Work out the finished part from the listing and answer in its coordinate system (mm). Face numbers are marked on the shaded views. A direction names the side the tool comes from. Give positions to 0.01 mm unless a question says otherwise; leave off trailing zeros. Write each loop counter-clockwise with the first axis right and the second up, starting at its lowest first coordinate (ties: lowest second). Pieces come first, ordered by that corner, then holes. Notation, with made-up numbers: (38, 40) -> (85, 40) arc R27 ccw to (85, 62) -> close; hole circle Ø6 at (12, 15.25). An arc over 180 degrees is marked (long way). Write item = value, one per line. Start each with the question number.
from build123d import *

# Parameters (mm, degrees)
SKETCH1_W           = 25.4
SKETCH1_H           = 50.8
SKETCH1_W_2         = 20.32
SKETCH1_H_2         = 45.72
BOSS_EXTRUDE1_DEPTH = 139.7
SKETCH2_R           = 2.032
CUT_EXTRUDE1_DEPTH  = 150.191219581
SKETCH3_R           = 2.032
SKETCH3_R_2         = 14.605
SKETCH3_R_3         = 3.302
CUT_EXTRUDE2_DEPTH  = 145.244271983


with BuildPart() as part:
    # Sketch1 → Boss-Extrude1 (new body)
    with BuildSketch(Plane.XY):
        Rectangle(SKETCH1_W, SKETCH1_H)
        Rectangle(SKETCH1_W_2, SKETCH1_H_2, mode=Mode.SUBTRACT)
    extrude(amount=BOSS_EXTRUDE1_DEPTH)

    # Sketch2 → Cut-Extrude1 (cut, through all)
    with BuildSketch(Plane(origin=(0, 25.4, 0), x_dir=(1, 0, 0), z_dir=(0, 1, 0))):
        Circle(SKETCH2_R)
        with Locations(Location((0, -25.4, 0), (0, 0, 270))):
            Circle(SKETCH2_R)
        with Locations(Location((0, -50.8, 0), (0, 0, 270))):
            Circle(SKETCH2_R)
        with Locations(Location((0, -76.2, 0), (0, 0, 270))):
            Circle(SKETCH2_R)
        with Locations(Location((0, -101.6, 0), (0, 0, 270))):
            Circle(SKETCH2_R)
        with Locations(Location((0, -127, 0), (0, 0, 270))):
            Circle(SKETCH2_R)
        with Locations((0, -152.4)):
            Circle(SKETCH2_R)
        with Locations((0, -177.8)):
            Circle(SKETCH2_R)
        with Locations((0, -203.2)):
            Circle(SKETCH2_R)
        with Locations((0, -228.6)):
            Circle(SKETCH2_R)
    extrude(amount=-CUT_EXTRUDE1_DEPTH, mode=Mode.SUBTRACT)

    # Sketch3 → Cut-Extrude2 (cut, through all)
    with BuildSketch(Plane.ZY.offset(12.7)):
        with Locations((133.35, 19.05)):
            Circle(SKETCH3_R)
        with Locations((95.25, -19.05)):
            Circle(SKETCH3_R)
        with Locations((114.3, 0)):
            Circle(SKETCH3_R_2)
        with Locations((12.7, 12.7)):
            Circle(SKETCH3_R_3)
        with Locations((38.1, 12.7)):
            Circle(SKETCH3_R_3)
        with Locations((38.1, -12.7)):
            Circle(SKETCH3_R_3)
        with Locations((12.7, -12.7)):
            Circle(SKETCH3_R_3)
    extrude(amount=-CUT_EXTRUDE2_DEPTH, mode=Mode.SUBTRACT)


solid = part.part
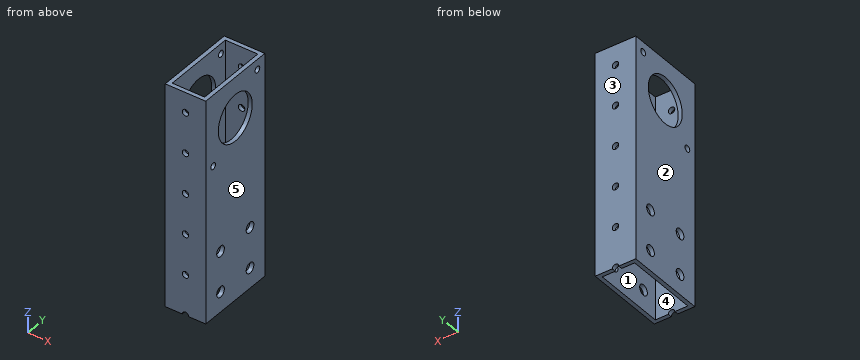
(1) Determine the mould class of the marked faces 1, 2 and 3 for opening direction X: pulls with the +X half, pulls with the -X half, needs draft (parallel to the pull), parting line crosses it, or undercut.
(2) A cutting plane is placed at D-D, the plane y = -19.05. Write down the section's boundary in (x, z), then the cut area to 3 significant figures.
(3) A cutting plane is placed at B-B, the plane z = 95.25. Write down the section's boundary in (x, y).
(4) A cutting plane is placed at C-C, the plane z = 12.7. Write down the section's boundary in (x, y).
(5) A cutting plane is placed at A-A, the plane y = 0. Write down the section's boundary in (x, z) (3 decimals), then the cut area to 3 significant figures.
(6) For the marked faces 4 and 5, determine the directions among +Z, -Z, +X, -X, +Y, -Y from which every point of the face is accessible in a straight line to the end or side of a thin tool.
(7) Find the intervals of material crossed by line 1 along Y through (x, z) = (-11.1, 38.1); line 2 along X through (y, z) = (1, 129); line 3 along Y through (x, z) = (-7.25, 133.5), in increasing order.
Results list:
q1.face_1 = undercut
q1.face_2 = pulls with the -X half
q1.face_3 = needs draft
q2.outline = (-12.7, 0) -> (-10.16, 0) -> (-10.16, 93.22) -> (-12.7, 93.22) -> close; (-12.7, 97.28) -> (-10.16, 97.28) -> (-10.16, 139.7) -> (-12.7, 139.7) -> close; (10.16, 0) -> (12.7, 0) -> (12.7, 93.22) -> (10.16, 93.22) -> close; (10.16, 97.28) -> (12.7, 97.28) -> (12.7, 139.7) -> (10.16, 139.7) -> close
q2.area = 689 mm²
q3.outline = (-12.7, -25.4) -> (12.7, -25.4) -> (12.7, -21.08) -> (10.16, -21.08) -> (10.16, -22.86) -> (-10.16, -22.86) -> (-10.16, -21.08) -> (-12.7, -21.08) -> close; (-12.7, -17.02) -> (-10.16, -17.02) -> (-10.16, 22.86) -> (10.16, 22.86) -> (10.16, -17.02) -> (12.7, -17.02) -> (12.7, 25.4) -> (-12.7, 25.4) -> close
q4.outline = (-12.7, -25.4) -> (12.7, -25.4) -> (12.7, -16) -> (10.16, -16) -> (10.16, -22.86) -> (-10.16, -22.86) -> (-10.16, -16) -> (-12.7, -16) -> close; (-12.7, -9.4) -> (-10.16, -9.4) -> (-10.16, 9.4) -> (-12.7, 9.4) -> close; (-12.7, 16) -> (-10.16, 16) -> (-10.16, 22.86) -> (10.16, 22.86) -> (10.16, 16) -> (12.7, 16) -> (12.7, 25.4) -> (-12.7, 25.4) -> close; (10.16, -9.4) -> (12.7, -9.4) -> (12.7, 9.4) -> (10.16, 9.4) -> close
q5.outline = (-12.7, 0) -> (-10.16, 0) -> (-10.16, 99.695) -> (-12.7, 99.695) -> close; (-12.7, 128.905) -> (-10.16, 128.905) -> (-10.16, 139.7) -> (-12.7, 139.7) -> close; (10.16, 0) -> (12.7, 0) -> (12.7, 99.695) -> (10.16, 99.695) -> close; (10.16, 128.905) -> (12.7, 128.905) -> (12.7, 139.7) -> (10.16, 139.7) -> close
q5.area = 561 mm²
q6.face_4 = +Z, -Z
q6.face_5 = +Z, -Z, +X, +Y, -Y
q7.line_1 = -25.4 to -16, -9.4 to 9.4, 16 to 25.4
q7.line_2 = -12.7 to -10.16, 10.16 to 12.7
q7.line_3 = -25.4 to -22.86, 22.86 to 25.4
